Model file for the job. Use its own axes, mm. A direction names the side the tool comes from. Round coordinates to 2 decimals unless told otherwise and drop trailing zeros. Order: outer loops, then holes, each group sorted by start corner. A loop starts at its lowest first (then second) coordinate and runs counter-clockwise, first axis right, second up. Notation, with made-up numbers: (25.5, 51.25) -> (40.5, 51.25) arc R22 ccw to (40.5, 71.25) -> close; hole circle Ø11 at (18, 53.5). An arc over 180 degrees is marked (long way). Put each result on its own line as item: value. Start each with the question number.
Q1. Cut at D-D, the plane x = -47. List the corners of the cut face in (y, z) (3 decimals), and give its area (3 significant figures).
Q2. Cut at C-C, the plane z = 47. State how many separate pieces and enclosed holes the cut face has, and give its area (3 significant figures).
Q3. Cut at A-A, the plane y = -33. List the corners of the cut face in (x, z) (3 decimals).
Q4. Cut at B-B, the plane x = -33.02. List the corners of the cut face in (y, z) (3 decimals), and give its area (3 significant figures).
Q5. 3-axis set-ups, long thin cutter, end or side, ignore diameter. For faces 4 (the face through (-33, -41.275, 27)), 5 (the face through (-5.45, 23.82, 1.59)), 6 (the face through (-44.79, 24.17, 21.12)), 7 (the face through (-45, 22.606, 5)), 8 (the face through (-20.96, 39.464, 26.923)): which of +Z, -Z, +X, -X, +Y, -Y reach the whole face in a straight line?
Q6. Pull direction Y, two halves, no side cores. Call faces 1 (the face through (-51.054, -34, 16)), 2 (the face through (-26, -56.134, 27)), 3 (the face through (-44.196, -33, 16)): released by +Y, released by -Y, zero draft, split by the parting line, or undercut.
Q7. Probe L1, parallel to Y at x = -34, z = 5 (3 decimals); L2, parallel to Z at x = -33, y = -52; L3, parallel to Y at x = -14, z = 10. List the from-to ranges inside material, lowest first.
Q8. Flat gauge pins, fed straight in: P1, Ø3.5, axis at y = 49, z = 42.5, coming from the -X side; P2, Ø11, axis at x = -47, z = 4, coming from the +Y side; P3, Ø12, axis at y = -6, z = 46, coming from the -X side. Where does each tip first touch, or does it go through?
from build123d import *

# Parameters (mm, degrees)
EXTRUDE1_DEPTH                                = 54.61
SKETCH6_R                                     = 3.96875
SKETCH6_W                                     = 6.858
SKETCH6_H                                     = 22.225
CUT_EXTRUDE1_DEPTH                            = 113.268
SKETCH8_W                                     = 6.35
SKETCH8_H                                     = 18.669
CUT_EXTRUDE2_DEPTH                            = 23.225
SKETCH13_R                                    = 23.8125
EXTRUDE4_DEPTH                                = 33.02
FILLET1_R                                     = 6.35
CBORE_FOR_1_4_SOCKET_HEAD_CAP_SCREW1_AT_COUNT = 2
CBORE_FOR_1_4_SOCKET_HEAD_CAP_SCREW1_AT_PITCH = 53.975
CHAMFER4_SIZE                                 = 10.16
CHAMFER7_SIZE                                 = 15.875
F_1_4_0_25_DIAMETER_HOLE1_D                   = 6.35
EXTRUDE9_DEPTH                                = 32.385
EXTRUDE8_DEPTH                                = 17.62


with BuildPart() as part:
    # Sketch5 → Extrude1 (new body)
    with BuildSketch(Plane.XY):
        with BuildLine():
            Line((0, -56.134), (0, 56.134))
            Line((0, 56.134), (-40.894, 56.134))
            Line((-40.894, 56.134), (-51.054, 45.974))
            Line((-51.054, 45.974), (-51.054, 22.606))
            Line((-51.054, 22.606), (-44.196, 22.606))
            Line((-44.196, 22.606), (-44.196, 34.925))
            ThreePointArc((-44.196, 34.925), (-42.336128061, 39.415128061), (-37.846, 41.275))
            Line((-37.846, 41.275), (-25.4, 41.275))
            ThreePointArc((-25.4, 41.275), (-20.909871939, 39.415128061), (-19.05, 34.925))
            Line((-19.05, 34.925), (-19.05, -34.925))
            ThreePointArc((-19.05, -34.925), (-20.909871939, -39.415128061), (-25.4, -41.275))
            Line((-25.4, -41.275), (-37.846, -41.275))
            ThreePointArc((-37.846, -41.275), (-42.336128061, -39.415128061), (-44.196, -34.925))
            Line((-44.196, -34.925), (-44.196, -22.606))
            Line((-44.196, -22.606), (-51.054, -22.606))
            Line((-51.054, -22.606), (-51.054, -45.974))
            Line((-51.054, -45.974), (-40.894, -56.134))
            Line((-40.894, -56.134), (0, -56.134))
        make_face()
    extrude(amount=EXTRUDE1_DEPTH)

    # Sketch6 → Cut-Extrude1 (cut, through all)
    with BuildSketch(Plane.XZ.offset(56.134)):
        with Locations(Location((-33.02, 44.5008, 0), (0, 0, 270))):  # turned: the seam where the file's is
            Circle(SKETCH6_R)
        with Locations((-47.625, 43.4975)):
            Rectangle(SKETCH6_W, SKETCH6_H)
    extrude(amount=-CUT_EXTRUDE1_DEPTH, mode=Mode.SUBTRACT)

    # Sketch8 → Cut-Extrude2 (cut, through all)
    with BuildSketch(Plane.XY.offset(32.385)):
        with Locations((-41.021, -31.9405)):
            Rectangle(SKETCH8_W, SKETCH8_H)
        with BuildLine():
            Line((-44.196, 34.925), (-44.196, 41.275))
            Line((-44.196, 41.275), (-37.846, 41.275))
            ThreePointArc((-37.846, 41.275), (-42.336128061, 39.415128061), (-44.196, 34.925))
        make_face()
    extrude(amount=CUT_EXTRUDE2_DEPTH, mode=Mode.SUBTRACT)

    # Sketch13 → Extrude4 (cut)
    with BuildSketch(Plane(origin=(0, 0, 0), x_dir=(-1, 0, 0), z_dir=(0, 0, -1))):
        with Locations((34.544, 0)):
            Circle(SKETCH13_R)
    extrude(amount=-EXTRUDE4_DEPTH, mode=Mode.SUBTRACT)

    # Fillet1
    fillet1_edges = [part.edges().sort_by_distance(p)[0] for p in [
        (-19.05, -18.082342775, 16.51),
        (-19.05, 18.082342775, 16.51),
    ]]
    fillet(fillet1_edges, radius=FILLET1_R)

    # Sketch18 → CBORE for 1/4 Socket Head Cap Screw1 (revolve, cut)
    with BuildSketch(Plane(origin=(-7.874, 26.9875, 0), x_dir=(0, 1, 0), z_dir=(1, 0, 0))):
        Polygon((0, 0), (0, 21.434665582), (3.96875, 19.05), (3.96875, 2.8448), (3.9878, 2.8448), (3.9878, 0.3683), (4.3561, 0), align=None)
    cbore_for_1_4_socket_head_cap_screw1 = revolve(axis=Axis((-7.874, 26.9875, -6.35), (0, 0, 1)), mode=Mode.SUBTRACT)

    # CBORE for 1/4 Socket Head Cap Screw1 at: CBORE for 1/4 Socket Head Cap Screw1 ×2
    with Locations(*[(0, -i * CBORE_FOR_1_4_SOCKET_HEAD_CAP_SCREW1_AT_PITCH, 0) for i in range(1, CBORE_FOR_1_4_SOCKET_HEAD_CAP_SCREW1_AT_COUNT)]):
        add(cbore_for_1_4_socket_head_cap_screw1, mode=Mode.SUBTRACT)

    # Chamfer4
    chamfer4_edges = [part.edges().sort_by_distance(p)[0] for p in [
        (0, 56.134, 27.305),
        (0, -56.134, 27.305),
    ]]
    chamfer(chamfer4_edges, length=CHAMFER4_SIZE)

    # Chamfer7
    chamfer7_edges = [part.edges().sort_by_distance(p)[0] for p in [
        (0, 0, 54.61),
    ]]
    chamfer(chamfer7_edges, length=CHAMFER7_SIZE)

    # 1/4 (0.25) Diameter Hole1 (through all)
    with Locations(Plane(origin=(0, 0, 0), x_dir=(-1, 0, 0), z_dir=(0, 0, -1))):
        with Locations((7.874, 26.9875), (7.874, -26.9875)):
            Hole(F_1_4_0_25_DIAMETER_HOLE1_D / 2)

    # Sketch22 → Extrude9 (add)
    with BuildSketch(Plane(origin=(0, 0, 0), x_dir=(-1, 0, 0), z_dir=(0, 0, -1))):
        with BuildLine():
            Line((38.354, -24.765), (38.354, -22.606))
            Line((38.354, -22.606), (44.196, -22.606))
            Line((44.196, -22.606), (44.196, -31.094647384))
            ThreePointArc((44.196, -31.094647384), (42.51227796, -26.787867844), (38.354, -24.765))
        make_face()
    extrude9 = extrude(amount=-EXTRUDE9_DEPTH)

    # Mirror3: Extrude9 across plane
    add(extrude9.mirror(Plane.ZX))

    # Sketch17 → Extrude8 (cut)
    with BuildSketch(Plane.ZY.offset(51.054)):
        Polygon((32.385, -25.781), (32.385, -22.606), (10.16, -22.606), align=None)
        Polygon((32.385, 25.781), (32.385, 22.606), (10.16, 22.606), align=None)
    extrude(amount=-EXTRUDE8_DEPTH, mode=Mode.SUBTRACT)


solid = part.part
Ans:
1. outline: (-50.028, 0) -> (-22.606, 0) -> (-22.606, 10.16) -> (-25.781, 32.385) -> (-50.028, 32.385) -> close; (22.606, 0) -> (50.028, 0) -> (50.028, 32.385) -> (25.781, 32.385) -> (22.606, 10.16) -> close
1. area: 1,710 mm^2
2. separate pieces: 3
2. enclosed holes: 0
2. area: 1,750 mm^2
3. outline: (-51.054, 0) -> (-44.196, 0) -> (-44.196, 32.385) -> (-51.054, 32.385) -> close; (-19.05, 0) -> (0, 0) -> (0, 38.735) -> (-15.875, 54.61) -> (-19.05, 54.61) -> close
4. outline: (-56.134, 0) -> (-41.275, 0) -> (-41.275, 40.532) -> (-56.134, 40.532) -> close; (-56.134, 48.47) -> (-41.275, 48.47) -> (-41.275, 54.61) -> (-56.134, 54.61) -> close; (41.275, 0) -> (56.134, 0) -> (56.134, 40.532) -> (41.275, 40.532) -> close; (41.275, 48.47) -> (56.134, 48.47) -> (56.134, 54.61) -> (41.275, 54.61) -> close
4. area: 1,390 mm^2
5. face 4: +Z
5. face 5: -Z
5. face 6: +Z, -X
5. face 7: +Z, -Z, -X
5. face 8: +Z, -Z
6. face 1: zero draft
6. face 2: released by -Y
6. face 3: undercut
7. L1: y = -56.134 to -41.275, 41.275 to 56.134
7. L2: z = 0 to 40.53, 48.47 to 54.61
7. L3: y = -56.13 to -12.04, 12.04 to 56.13
8. P1: stops at x = -44.2
8. P2: stops at y = 55.53
8. P3: stops at x = -19.05
